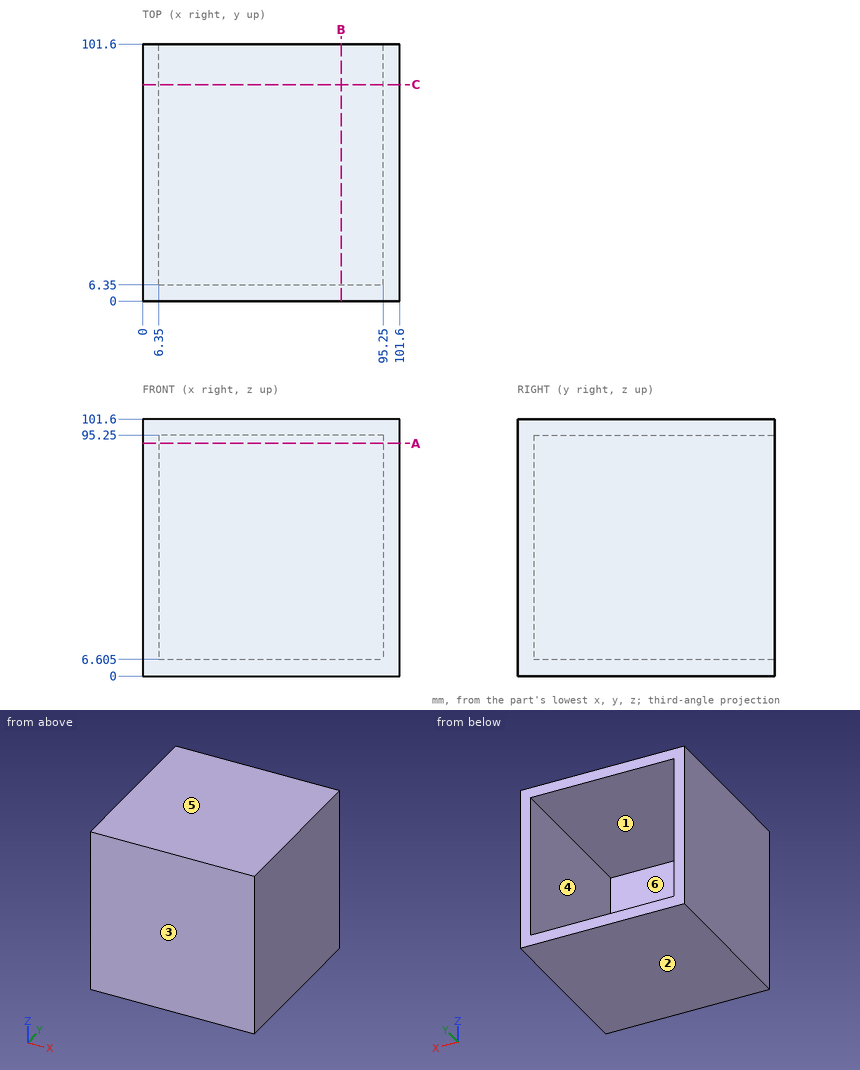
Design review of the part shown in the three views and the two pictorial views. Dimensions are in mm from the part's minimum x, y and z. A direction names the side the tool comes from. Give positions to 0.01 mm unless a question says otherwise; leave off trailing zeros. Order: outer loops, then holes, each group sorted by start corner. A loop starts at its lowest first (then second) coordinate and runs counter-clockwise, first axis right, second up. Notation, with made-up numbers: (9.5, -21.5) -> (65.5, -21.5) arc R35 ccw to (65.5, 11.5) -> close; hole circle Ø10 at (79, -3.5). An arc over 180 degrees is marked (long way). Write each question's results on one line, items separated by ' | '. Start each with the question number.
Q1. For pin 1 (1.5 mm diameter, centred on x = 56.5, z = 62.5, fed in from +Y); pin 2 (12 mm diameter, centred on x = 37, z = 71, fed in from -Y), all flat-tipped, find the tip position at first contact; note any pin that passes through.
Q2. Add section B-B on x = 78.5. Give the boundary of the cut face in (y, z) (3 decimals).
Q3. Add section A-A on z = 92. Give the boundary of the cut face in (x, y), and give its area (3 significant figures).
Q4. Mouldability with a two-part tool opening along Z and no side actions: class the marked faces 3, 4, 5 and 6 as +Z half, -Z half, draft (parallel to the pull), parting line (faces both ways), or undercut.
Q5. Add section C-C on y = 85.5. Give the boundary of the cut face in (x, z) (3 decimals).
Q6. Machinability: for the marked faces 1 and 2, which of the approach directions +Z, -Z, +X, -X, +Y, -Y give a long, thin tool a straight path to every point of the face, cutting with its end or side? Answer none if there is none.
Q7. Wall thickness on L1, parallel to X at y = 56, z = 59.5; L2, parallel to Z at x = 74, y = 90 (3 decimals); L3, parallel to Y at x = 59.5, z = 58: over which ranges is each line inside the solid? List them lowest first. Write a range as from..to.
Found:
1) pin 1: stops at y = 6.35 | pin 2: stops at y = 0
2) outline: (0, 0) -> (101.6, 0) -> (101.6, 6.605) -> (6.35, 6.605) -> (6.35, 95.25) -> (101.6, 95.25) -> (101.6, 101.6) -> (0, 101.6) -> close
3) outline: (0, 0) -> (101.6, 0) -> (101.6, 101.6) -> (95.25, 101.6) -> (95.25, 6.35) -> (6.35, 6.35) -> (6.35, 101.6) -> (0, 101.6) -> close | area: 1,850 mm2
4) face 3: draft | face 4: undercut | face 5: +Z half | face 6: undercut
5) outline: (0, 0) -> (101.6, 0) -> (101.6, 101.6) -> (0, 101.6) -> close; hole (6.35, 6.605) -> (95.25, 6.605) -> (95.25, 95.25) -> (6.35, 95.25) -> close
6) face 1: +Y | face 2: -Z, +X, -X, +Y, -Y
7) L1: x = 0..6.35, 95.25..101.6 | L2: z = 0..6.605, 95.25..101.6 | L3: y = 0..6.35
